```python
from build123d import *

# Parameters (mm, degrees)
BOSS_EXTRUDE1_DEPTH            = 2.5
BOSS_EXTRUDE2_START            = 2.5
BOSS_EXTRUDE2_DEPTH            = 30
SKETCH1_5_R                    = 3
BOSS_EXTRUDE4_DEPTH            = 30
CUT_EXTRUDE3_REACH             = 134.823
SKETCH8_W                      = 2
SKETCH8_H                      = 20
CUT_EXTRUDE3_DIRECTION_2_REACH = 134.823
LPATTERN1_START                = 6.25
LPATTERN1_DEPTH                = 20


# Read off the part's stored shape, not the designer's step: LPattern1
with BuildPart() as part:
    # Sketch1 → Boss-Extrude1 (new body)
    with BuildSketch(Plane(origin=(0, 0, 0), x_dir=(1, 0, 0), z_dir=(0, 1, 0))):
        with BuildLine():
            Line((-30, 70), (30, 70))
            ThreePointArc((30, 70), (37.071067812, 67.071067812), (40, 60))
            Line((40, 60), (40, -60))
            ThreePointArc((40, -60), (37.071067812, -67.071067812), (30, -70))
            Line((30, -70), (-30, -70))
            ThreePointArc((-30, -70), (-37.071067812, -67.071067812), (-40, -60))
            Line((-40, -60), (-40, 60))
            ThreePointArc((-40, 60), (-37.071067812, 67.071067812), (-30, 70))
        make_face()
    extrude(amount=BOSS_EXTRUDE1_DEPTH)

    # Sketch1<3> → Boss-Extrude2 (add)
    with BuildSketch(Plane(origin=(0, 0, 0), x_dir=(1, 0, 0), z_dir=(0, 1, 0)).offset(BOSS_EXTRUDE2_START)):
        with BuildLine():
            Line((-30, 70), (30, 70))
            ThreePointArc((30, 70), (37.071067812, 67.071067812), (40, 60))
            Line((40, 60), (40, -60))
            ThreePointArc((40, -60), (37.071067812, -67.071067812), (30, -70))
            Line((30, -70), (-30, -70))
            ThreePointArc((-30, -70), (-37.071067812, -67.071067812), (-40, -60))
            Line((-40, -60), (-40, 60))
            ThreePointArc((-40, 60), (-37.071067812, 67.071067812), (-30, 70))
        make_face()
        with BuildLine():
            Line((-37, 60), (-37, -60))
            ThreePointArc((-37, -60), (-34.949747468, -64.949747468), (-30, -67))
            Line((-30, -67), (30, -67))
            ThreePointArc((30, -67), (34.949747468, -64.949747468), (37, -60))
            Line((37, -60), (37, 60))
            ThreePointArc((37, 60), (34.949747468, 64.949747468), (30, 67))
            Line((30, 67), (-30, 67))
            ThreePointArc((-30, 67), (-34.949747468, 64.949747468), (-37, 60))
        make_face(mode=Mode.SUBTRACT)
    extrude(amount=BOSS_EXTRUDE2_DEPTH)

    # Sketch1<5> → Boss-Extrude4 (add)
    with BuildSketch(Plane(origin=(0, 0, 0), x_dir=(1, 0, 0), z_dir=(0, 1, 0))):
        with Locations(Location((27, -57, 0), (0, 0, 270))):
            Circle(SKETCH1_5_R)
        with Locations(Location((-27, -57, 0), (0, 0, 90))):
            Circle(SKETCH1_5_R)
        with Locations(Location((-27, 57, 0), (0, 0, 270))):
            Circle(SKETCH1_5_R)
        with Locations(Location((27, 57, 0), (0, 0, 90))):
            Circle(SKETCH1_5_R)
    extrude(amount=BOSS_EXTRUDE4_DEPTH)

    # Sketch8 → Cut-Extrude3 (cut, up to next)
    with BuildSketch(Plane(origin=(37, 16.25, -37), x_dir=(0.7071067811865538, 0, 0.7071067811865412), z_dir=(-0.7071067811865412, 0, 0.7071067811865538)), mode=Mode.PRIVATE) as cut_extrude3_sk1:
        Rectangle(SKETCH8_W, SKETCH8_H)
    cut_extrude3_tool1 = extrude(cut_extrude3_sk1.sketch, amount=-CUT_EXTRUDE3_REACH, mode=Mode.PRIVATE) & part.part
    cut_extrude3 = cut_extrude3_tool1.solids().sort_by_distance((37, 16.25, -37))[0]
    add(cut_extrude3, mode=Mode.SUBTRACT)

    # Sketch8 → Cut-Extrude3 direction 2 (cut, up to next)
    with BuildSketch(Plane(origin=(37, 16.25, -37), x_dir=(0.7071067811865538, 0, 0.7071067811865412), z_dir=(-0.7071067811865412, 0, 0.7071067811865538)), mode=Mode.PRIVATE) as cut_extrude3_direction_2_sk1:
        Rectangle(SKETCH8_W, SKETCH8_H)
    cut_extrude3_direction_2_tool1 = extrude(cut_extrude3_direction_2_sk1.sketch, amount=CUT_EXTRUDE3_DIRECTION_2_REACH, mode=Mode.PRIVATE) & part.part
    cut_extrude3_direction_2 = cut_extrude3_direction_2_tool1.solids().sort_by_distance((37, 16.25, -37))[0]
    add(cut_extrude3_direction_2, mode=Mode.SUBTRACT)

    # LPattern1 outline → LPattern1 (cut)
    with BuildSketch(Plane(origin=(0, 0, 0), x_dir=(1, 0, 0), z_dir=(0, 1, 0)).offset(LPATTERN1_START)):
        Polygon((37, -42.414213562), (40, -39.414213562), (40, -36.585786438), (37, -39.585786438), align=None)
        Polygon((37, -36.414213562), (40, -33.414213562), (40, -30.585786438), (37, -33.585786438), align=None)
        Polygon((37, -30.414213562), (40, -27.414213562), (40, -24.585786438), (37, -27.585786438), align=None)
        Polygon((37, -24.414213562), (40, -21.414213562), (40, -18.585786438), (37, -21.585786438), align=None)
        Polygon((37, -18.414213562), (40, -15.414213562), (40, -12.585786438), (37, -15.585786438), align=None)
        Polygon((37, -12.414213562), (40, -9.414213562), (40, -6.585786438), (37, -9.585786438), align=None)
        Polygon((37, -6.414213562), (40, -3.414213562), (40, -0.585786438), (37, -3.585786438), align=None)
        Polygon((37, -0.414213562), (40, 2.585786438), (40, 5.414213562), (37, 2.414213562), align=None)
        Polygon((37, 5.585786438), (40, 8.585786438), (40, 11.414213562), (37, 8.414213562), align=None)
        Polygon((37, 11.585786438), (40, 14.585786438), (40, 17.414213562), (37, 14.414213562), align=None)
        Polygon((37, 17.585786438), (40, 20.585786438), (40, 23.414213562), (37, 20.414213562), align=None)
        Polygon((37, 23.585786438), (40, 26.585786438), (40, 29.414213562), (37, 26.414213562), align=None)
        Polygon((37, 29.585786438), (40, 32.585786438), (40, 35.414213562), (37, 32.414213562), align=None)
    lpattern1 = extrude(amount=LPATTERN1_DEPTH, mode=Mode.SUBTRACT)

    # Mirror2: Cut-Extrude3, Cut-Extrude3 direction 2, LPattern1 across plane
    add(cut_extrude3.mirror(Plane(origin=(0, 0, 0), x_dir=(0, 0, 1), z_dir=(1, 0, 0))), mode=Mode.SUBTRACT)
    add(cut_extrude3_direction_2.mirror(Plane(origin=(0, 0, 0), x_dir=(0, 0, 1), z_dir=(1, 0, 0))), mode=Mode.SUBTRACT)
    add(lpattern1.mirror(Plane(origin=(0, 0, 0), x_dir=(0, 0, 1), z_dir=(1, 0, 0))), mode=Mode.SUBTRACT)


solid = part.part
```
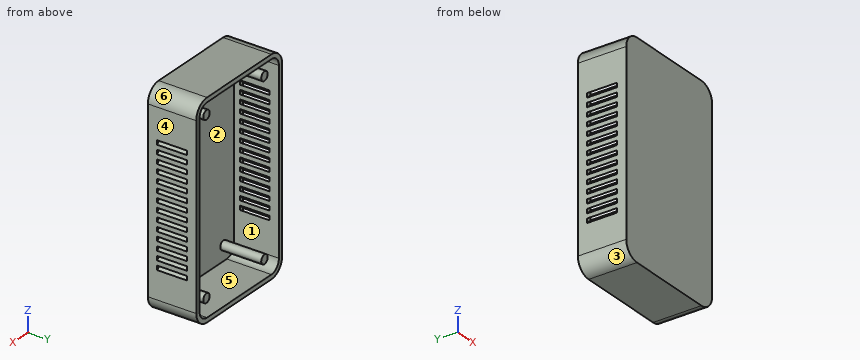
Geometry: final body of the model. Coordinates: model frame, mm. Face numbers are marked on the shaded views. A direction names the side the tool comes from. Coordinates: 2 decimals unless noted, no trailing zeros. Order: outer loops, then holes, each group sorted by start corner. A loop starts at its lowest first (then second) coordinate and runs counter-clockwise, first axis right, second up.
Item 1: Draft query along Z for the marked faces 1, 2, 3 and 4. Return one class per face: released by +Z, released by -Z, zero draft, split by the parting line, or undercut.
Answer:
face 1: undercut
face 2: undercut
face 3: released by -Z
face 4: zero draft
Item 2: Section query D-D (x = 16.5). Output: boundary loops of the cut face in (y, z), then the cut area to 3 significant figures.
Answer:
outline: (0, -70) - (32.5, -70) - (32.5, -67) - (2.5, -67) - (2.5, 67) - (32.5, 67) - (32.5, 70) - (0, 70) - close
area: 530 mm2
Item 3: Section query A-A (z = 57). Output: boundary loops of the cut face in (x, y).
Answer:
outline: (-40, 0) - (40, 0) - (40, 32.5) - (37, 32.5) - (37, 2.5) - (30, 2.5) - (30, 30) - (24, 30) - (24, 2.5) - (-24, 2.5) - (-24, 30) - (-30, 30) - (-30, 2.5) - (-37, 2.5) - (-37, 32.5) - (-40, 32.5) - close
Item 4: Section query C-C (x = -27). Output: boundary loops of the cut face in (y, z), then the cut area to 3 significant figures.
Answer:
outline: (0, -70) - (32.5, -70) - (32.5, -67) - (2.5, -67) - (2.5, -60) - (30, -60) - (30, -54) - (2.5, -54) - (2.5, 54) - (30, 54) - (30, 60) - (2.5, 60) - (2.5, 67) - (32.5, 67) - (32.5, 70) - (0, 70) - close
area: 860 mm2
Item 5: Section query B-B (y = 23). State how many separate pieces and enclosed holes the cut face has, then the cut area to 3 significant figures.
Answer:
separate pieces: 32
enclosed holes: 0
area: 1,120 mm2
Item 6: Contact query for flat-ended pins moving along their axis: P1, Ø3, axis at x = 27, z = 56.5, coming from the +Y side; P2, Ø10, axis at x = 24, z = -30, coming from the +Y side. Output: stop coordinate, or through.
Answer:
P1: stops at y = 30
P2: stops at y = 2.5
Item 7: Access query for the marked faces 5 and 6. Directions: +Z, -Z, +X, -X, +Y, -Y. A direction counts if a zero-diameter tool reaches every point of the face in a straight line with its end or side. Return the directions, or none.
Answer:
face 5: +Y
face 6: +Z, +X, +Y, -Y
Item 8: Material intervals for line 1 along Z through (x, y) = (16, 23); line 2 along X through (y, z) = (27, -47.5); line 3 along Z through (x, y) = (-24.5, 20), sorted ascending.
Answer:
line 1: z = -70 to -67, 67 to 70
line 2: x = -40 to -37, 37 to 40
line 3: z = -70 to -67, -58.66 to -55.34, 55.34 to 58.66, 67 to 70
